Check sheet for the modelled part. Datum: model origin and axes. Units: mm. A direction names the side the tool comes from. Round coordinates to 2 decimals unless told otherwise and drop trailing zeros. Loops run counter-clockwise (first coordinate to the right, second up) from the corner with the lowest first, then second, coordinate; pieces in that order, holes last. Notation, with made-up numbers: (-10.75, 10.5) - (1.25, 10.5) arc R23 cw to (1.25, 38.5) - close; hole circle Ø10 at (29, -5). An arc over 180 degrees is marked (long way). Put each result on its own line as item: value. Start each with the question number.
```python
from build123d import *

# Parameters (mm, degrees)
BOSS_EXTRUDE1_DEPTH = 3.5
SKETCH2_R           = 3.96875
SKETCH2_R_2         = 3
SKETCH2_R_3         = 3.54844416
CUT_EXTRUDE3_DEPTH  = 6


with BuildPart() as part:
    # Sketch1 → Boss-Extrude1 (new body)
    with BuildSketch(Plane(origin=(0, 0, 0), x_dir=(1, 0, 0), z_dir=(0, 1, 0))):
        with BuildLine():
            Line((-25, 60), (25, 60))
            ThreePointArc((25, 60), (32.071067812, 62.928932188), (35, 70))
            Line((35, 70), (35, 73))
            ThreePointArc((35, 73), (35.585786438, 74.414213562), (37, 75))
            Line((37, 75), (45, 75))
            ThreePointArc((45, 75), (48.535533906, 73.535533906), (50, 70))
            Line((50, 70), (50, -70))
            ThreePointArc((50, -70), (48.535533906, -73.535533906), (45, -75))
            Line((45, -75), (37, -75))
            ThreePointArc((37, -75), (35.585786438, -74.414213562), (35, -73))
            Line((35, -73), (35, -70))
            ThreePointArc((35, -70), (32.071067812, -62.928932188), (25, -60))
            Line((25, -60), (-25, -60))
            ThreePointArc((-25, -60), (-32.071067812, -62.928932188), (-35, -70))
            Line((-35, -70), (-35, -73))
            ThreePointArc((-35, -73), (-35.585786438, -74.414213562), (-37, -75))
            Line((-37, -75), (-45, -75))
            ThreePointArc((-45, -75), (-48.535533906, -73.535533906), (-50, -70))
            Line((-50, -70), (-50, 70))
            ThreePointArc((-50, 70), (-48.535533906, 73.535533906), (-45, 75))
            Line((-45, 75), (-37, 75))
            ThreePointArc((-37, 75), (-35.585786438, 74.414213562), (-35, 73))
            Line((-35, 73), (-35, 70))
            ThreePointArc((-35, 70), (-32.071067812, 62.928932188), (-25, 60))
        make_face()
    extrude(amount=BOSS_EXTRUDE1_DEPTH)

    # Sketch2 → Cut-Extrude3 (cut)
    with BuildSketch(Plane.XZ):
        with Locations(Location((0, 0, 0), (0, 0, 270))):
            Circle(SKETCH2_R)
        with Locations(Location((42.5, -68, 0), (0, 0, 270))):
            Circle(SKETCH2_R_2)
        with Locations(Location((-42.5, -68, 0), (0, 0, 270))):
            Circle(SKETCH2_R_3)
        with Locations(Location((42.5, 68, 0), (0, 0, 270))):
            Circle(SKETCH2_R_2)
        with Locations(Location((-42.5, 68, 0), (0, 0, 270))):
            Circle(SKETCH2_R_3)
    extrude(amount=-CUT_EXTRUDE3_DEPTH, mode=Mode.SUBTRACT)


solid = part.part
```
Q1. Material ranges on line 1 (X direction, y = 2.2, z = 0); line 2 (Z direction, x = 41, y = 1.9); line 3 (X direction, y = 1.2, z = -68), recorded low to high. Write a range as from..to.
Q2. Cross-section at C-C on x = 0. Enter the section's corners in (y, z).
Q3. Depth check by flat-ended pin: pin 1 Ø0.9 at (y, z) = (2.5, 71) entering from -X; pin 2 Ø0.9 at (y, z) = (2, -71.5) entering from -X; pin 3 Ø1.8 at (x, y) = (2, 1) entering from -Z. Enter the tip coordinate at first touch or a pass-through.
Q4. Set-up check for faces 1 (the face through (-31.99, 1.73, 62.85)), 2 (the face through (35, 2, -71)), 3 (the face through (12, 3.5, -1)): record each of +Z, -Z, +X, -X, +Y, -Y from which the full face is reachable in a straight line by a thin tool's end or side.
Q5. Cross-section at D-D on x = -12. Enter the section's corners in (y, z), and give its area (3 significant figures).
Q6. Cross-section at A-A on z = -62. Enter the section's corners in (x, y).
Q7. Draft check along X on faces 4 (the face through (-48, 2, 74)), 5 (the face through (-35, 2, 71)), 6 (the face through (41, 2, 75)). Enter one of: +X half, -X half, draft (parallel to the pull), parting line (faces both ways), or undercut.
Q8. Cross-section at B-B on y = 2.3. State how many separate pieces and enclosed holes the cut face has, and give its area (3 significant figures).
Answer list:
1. line 1: x = -50..-3.97, 3.97..50
1. line 2: z = -75..-70.6, -65.4..65.4, 70.6..75
1. line 3: x = -50..-46.05, -38.95..-34.8, 34.8..39.5, 45.5..50
2. outline: (0, -60) - (3.5, -60) - (3.5, -3.97) - (0, -3.97) - close; (0, 3.97) - (3.5, 3.97) - (3.5, 60) - (0, 60) - close
3. pin 1: stops at x = -49.97
3. pin 2: stops at x = -49.89
3. pin 3: stops at z = -60
4. face 1: +Z, +Y, -Y
4. face 2: -Z, +Y, -Y
4. face 3: +Z, -Z, +X, -X, +Y
5. outline: (0, -60) - (3.5, -60) - (3.5, 60) - (0, 60) - close
5. area: 420 mm2
6. outline: (-50, 0) - (-31, 0) - (-31, 3.5) - (-50, 3.5) - close; (31, 0) - (50, 0) - (50, 3.5) - (31, 3.5) - close
7. face 4: -X half
7. face 5: undercut
7. face 6: draft
8. separate pieces: 1
8. enclosed holes: 5
8. area: 12,800 mm2
